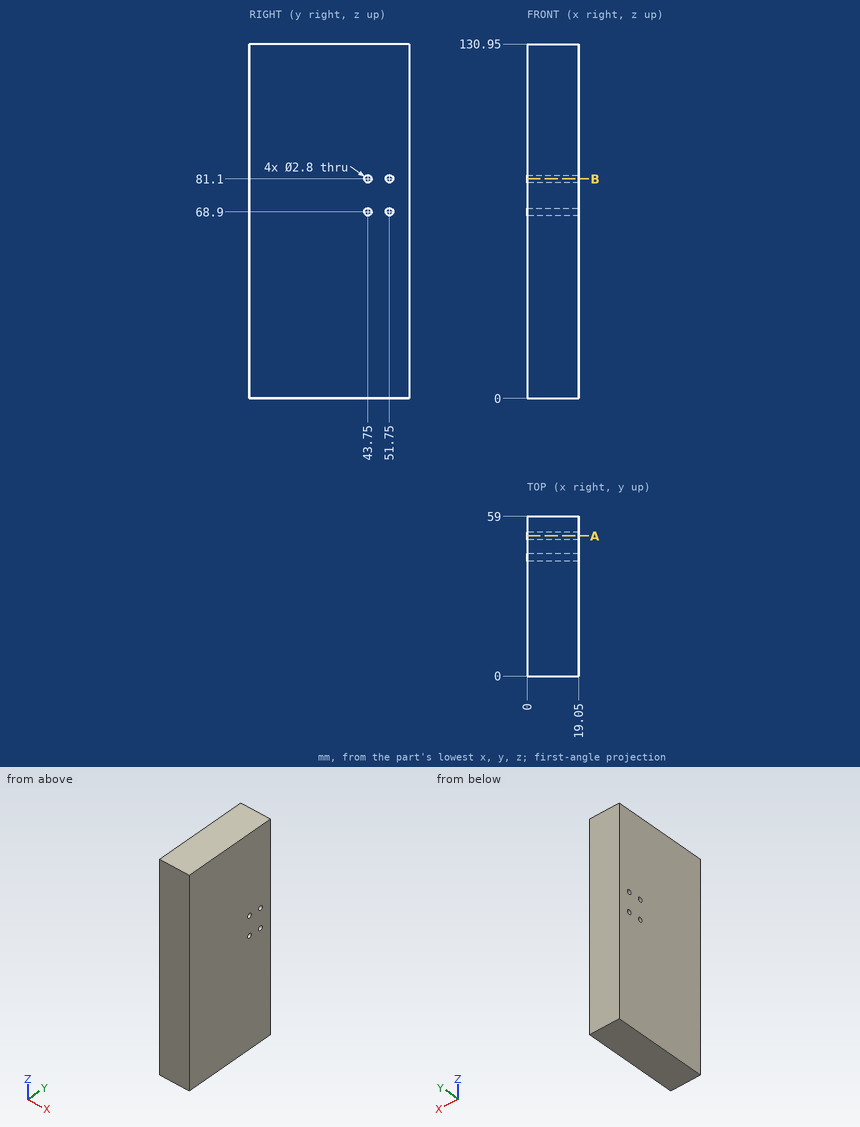
Geometry: see drawing. Coordinates: mm, zero at the bounding-box minimum. Coordinates: 2 decimals unless noted, no trailing zeros. Loops run counter-clockwise (first coordinate to the right, second up) from the corner with the lowest first, then second, coordinate; pieces in that order, holes last. Notation, with made-up numbers: (87, 59.25) - (117, 59.25) arc R24 ccw to (117, 94.25) - close; hole circle Ø3 at (-24.75, 89.25). An arc over 180 degrees is marked (long way). Put each result on its own line as item: value. Start each with the question number.
Q1. Pin query (flat end, axial travel): pin 1 Ø2 at (y, z) = (51.75, 68.9) entering from -X (3 decimals). Return the tip coordinate at first contact, or that it passes through.
Q2. Cut plane A-A, the plane y = 51.75. Return loops of the section in (x, z), and give its area (3 significant figures).
Q3. Line query: line 1 (Y direction, x = 12, z = 68.9); line 2 (Z direction, x = 4, y = 52.5). Output: solid intervals per line, ascending.
Q4. Cut plane B-B, the plane z = 81.1. Return loops of the section in (x, y), and give its area (3 significant figures).
Filled sheet:
1. pin 1: through
2. outline: (0, 0) - (19.05, 0) - (19.05, 67.5) - (0, 67.5) - close; (0, 70.3) - (19.05, 70.3) - (19.05, 79.7) - (0, 79.7) - close; (0, 82.5) - (19.05, 82.5) - (19.05, 130.95) - (0, 130.95) - close
2. area: 2,390 mm²
3. line 1: 0 to 42.35, 45.15 to 50.35, 53.15 to 59
3. line 2: 0 to 67.72, 70.08 to 79.92, 82.28 to 130.95
4. outline: (0, 0) - (19.05, 0) - (19.05, 42.35) - (0, 42.35) - close; (0, 45.15) - (19.05, 45.15) - (19.05, 50.35) - (0, 50.35) - close; (0, 53.15) - (19.05, 53.15) - (19.05, 59) - (0, 59) - close
4. area: 1,020 mm²
